Work out the finished part from the listing and answer in its coordinate system (mm). A direction names the side the tool comes from. Give positions to 0.01 mm unless a question says otherwise; leave off trailing zeros. Order: outer loops, then holes, each group sorted by start corner. A loop starts at its lowest first (then second) coordinate and runs counter-clockwise, first axis right, second up. Notation, with made-up numbers: (3, 13) -> (33, 13) arc R18 cw to (33, 42) -> close; hole circle Ø1 at (-33.75, 76). An arc over 180 degrees is marked (long way). Answer as CSV lines item,"result". Start each with the question number.
1. A cutting plane is placed at C-C (z = 11.5). Give the vertices of the cut face in (x, y).
2. A cutting plane is placed at D-D (x = -22). Give the vertices of the cut face in (y, z), then the cut area to 3 significant figures.
3. Find the intervals of material crossed by L1, parallel to Y at x = -14, z = 8; L2, parallel to Y at x = -8, z = 4.5; L3, parallel to X at y = 72, z = 26, in increasing order.
4. For a pull along Z with two mould halves and no side action, classify faces 1 (the flat face through (-17, 69, 28.071)), 2 (the cylindrical face through (-21.06, 66.58, 28.62)), 3 (the flat face through (-17, 60, 0)), 4 (the flat face through (-0.962, 62, 20)) as released by +Z, released by -Z, zero draft, split by the parting line, or undercut.
5. For faces 5 (the flat face through (-17, 70.809, 31)), 6 (the flat face through (-17, 69, 29.321)), 7 (the flat face through (-17, 62.681, 3)), 8 (the flat face through (-17, 64, 31.75)), determine the directions among +Z, -Z, +X, -X, +Y, -Y from which every point of the face is accessible in a straight line to the end or side of a thin tool.
6. A cutting plane is placed at A-A (y = 67). Give the vertices of the cut face in (x, z).
7. Flat-ended cylindrical pins translate along their axes: pin 1 (1.9 mm diameter, centred on x = -17, z = 30.5, fed in from +Y); pin 2 (4 mm diameter, centred on x = -19.5, y = 71.5, fed in from -Z); pin 3 (7 mm diameter, centred on x = -11, z = 3, fed in from +Y); pin 4 (5 mm diameter, centred on y = 64.5, z = 19.5, fed in from -X). Find the tip coordinate at first contact, or state that the pin passes through.
8. A cutting plane is placed at B-B (x = -8.5). Give the vertices of the cut face in (y, z).
from build123d import *

# Parameters (mm, degrees)
SKETCH1_W           = 53.34
SKETCH1_H           = 152.4
SKETCH1_R           = 1
BOSS_EXTRUDE1_DEPTH = 6.35
SKETCH2_W           = 32.258
SKETCH2_H           = 6.35
BOSS_EXTRUDE2_DEPTH = 31.75
SKETCH3_W           = 32.258
SKETCH3_H           = 6.35
BOSS_EXTRUDE3_DEPTH = 12.7
CUT_EXTRUDE1_REACH  = 136.322
SKETCH4_R           = 12.573
SKETCH5_W           = 32.258
SKETCH5_H           = 2.671239047
SKETCH5_H_2         = 2.428760953
BOSS_EXTRUDE4_DEPTH = 7.62
FILLET1_R           = 5.08
SKETCH8_W           = 53.34
SKETCH8_H           = 152.4
CUT_EXTRUDE4_DEPTH  = 133.964296911
SKETCH9_W           = 32.258
SKETCH9_H           = 5.842
BOSS_EXTRUDE6_DEPTH = 6.35


with BuildPart() as part:
    # Sketch1 → Boss-Extrude1 (new body)
    with BuildSketch(Plane.XY):
        with Locations((-17.091445783, 46.760481928)):
            Rectangle(SKETCH1_W, SKETCH1_H)
        with Locations((-36.141445783, 69.620481928)):
            Circle(SKETCH1_R, mode=Mode.SUBTRACT)
        with Locations((-8.201445783, 69.620481928)):
            Circle(SKETCH1_R, mode=Mode.SUBTRACT)
        with Locations((-41.221445783, 121.690481928)):
            Circle(SKETCH1_R, mode=Mode.SUBTRACT)
        with Locations((7.038554217, 120.420481928)):
            Circle(SKETCH1_R, mode=Mode.SUBTRACT)
    extrude(amount=BOSS_EXTRUDE1_DEPTH)

    # Sketch2 → Boss-Extrude2 (add)
    with BuildSketch(Plane.XY):
        with Locations((-17.091445783, 60.014063864)):
            Rectangle(SKETCH2_W, SKETCH2_H)
    extrude(amount=BOSS_EXTRUDE2_DEPTH)

    # Sketch3 → Boss-Extrude3 (add)
    with BuildSketch(Plane(origin=(0, 63.189063864, 0), x_dir=(1, 0, 0), z_dir=(0, 1, 0))):
        with Locations((-17.091445783, -28.575)):
            Rectangle(SKETCH3_W, SKETCH3_H)
    extrude(amount=BOSS_EXTRUDE3_DEPTH)

    # Sketch4 → Cut-Extrude1 (cut, up to next)
    with BuildSketch(Plane.XY.offset(31.75), mode=Mode.PRIVATE) as cut_extrude1_sk1:
        with Locations((-17.091445783, 78.510481928)):
            Circle(SKETCH4_R)
    cut_extrude1_tool1 = extrude(cut_extrude1_sk1.sketch, amount=-CUT_EXTRUDE1_REACH, mode=Mode.PRIVATE) & part.part
    add(cut_extrude1_tool1.solids().sort_by_distance((-17.091446, 78.510482, 31.75))[0], mode=Mode.SUBTRACT)

    # Sketch5 → Boss-Extrude4 (add)
    with BuildSketch(Plane(origin=(0, 63.189063864, 0), x_dir=(1, 0, 0), z_dir=(0, 1, 0))):
        with Locations((-17.091445783, -26.735619524)):
            Rectangle(SKETCH5_W, SKETCH5_H)
        with Locations((-17.091445783, -30.535619524)):
            Rectangle(SKETCH5_W, SKETCH5_H_2)
    extrude(amount=BOSS_EXTRUDE4_DEPTH)

    # Fillet1
    fillet1_edges = [part.edges().sort_by_distance(p)[0] for p in [
        (-17.091445783, 63.189063864, 25.4),
    ]]
    fillet(fillet1_edges, radius=FILLET1_R)

    # Sketch8 → Cut-Extrude4 (cut, through all)
    with BuildSketch(Plane.XY.offset(6.35)):
        with Locations((-17.091445783, 46.760481928)):
            Rectangle(SKETCH8_W, SKETCH8_H)
    extrude(amount=-CUT_EXTRUDE4_DEPTH, mode=Mode.SUBTRACT)

    # Sketch9 → Boss-Extrude6 (add)
    with BuildSketch(Plane(origin=(0, 0, 6.35), x_dir=(-1, 0, 0), z_dir=(0, 0, -1))):
        with Locations((17.091445783, 59.760063864)):
            Rectangle(SKETCH9_W, SKETCH9_H)
    extrude(amount=BOSS_EXTRUDE6_DEPTH)


solid = part.part
Answer sheet:
1,outline,"(-33.22, 56.84) -> (-0.96, 56.84) -> (-0.96, 63.19) -> (-33.22, 63.19) -> close"
2,outline,"(56.84, 0) -> (62.68, 0) -> (62.68, 6.35) -> (63.19, 6.35) -> (63.19, 20.32) arc R5.08 cw to (68.27, 25.4) -> (70.81, 25.4) -> (70.81, 28.07) -> (66.94, 28.07) -> (66.94, 29.32) -> (70.81, 29.32) -> (70.81, 31.75) -> (56.84, 31.75) -> close"
2,area,"247 mm^2"
3,L1,"y = 56.84 to 63.19"
3,L2,"y = 56.84 to 62.68"
3,L3,"x = -33.22 to -27.85, -6.34 to -0.96"
4,face 1,"undercut"
4,face 2,"undercut"
4,face 3,"released by -Z"
4,face 4,"zero draft"
5,face 5,"+Z, -Z, +Y"
5,face 6,"+Y"
5,face 7,"-Z, +X, -X, +Y"
5,face 8,"+Z, +X, -X, +Y, -Y"
6,outline,"(-33.22, 25.24) -> (-0.96, 25.24) -> (-0.96, 31.75) -> (-33.22, 31.75) -> close; hole (-22.15, 28.07) -> (-12.03, 28.07) -> (-12.03, 29.32) -> (-22.15, 29.32) -> close"
7,pin 1,"stops at y = 70.81"
7,pin 2,"stops at z = 25.4"
7,pin 3,"stops at y = 63.19"
7,pin 4,"stops at x = -33.22"
8,outline,"(56.84, 0) -> (62.68, 0) -> (62.68, 6.35) -> (63.19, 6.35) -> (63.19, 20.32) arc R5.08 cw to (68.27, 25.4) -> (70.81, 25.4) -> (70.81, 28.07) -> (69.33, 28.07) -> (69.33, 29.32) -> (70.81, 29.32) -> (70.81, 31.75) -> (56.84, 31.75) -> close"
